For this review, take the finished solid that the model builds, in its own axes (mm). Face numbers are marked on the shaded views. A direction names the side the tool comes from. Round coordinates to 2 decimals unless told otherwise and drop trailing zeros. Loops run counter-clockwise (first coordinate to the right, second up) from the corner with the lowest first, then second, coordinate; pieces in that order, holes last.
1. Consider section A-A on y = -58.5. State the section outline as (x, z) points (3 decimals), then the cut area to 3 significant figures.
2. Tool access review of the marked faces 1 and 2: name each direction out of +Z, -Z, +X, -X, +Y, -Y from which nothing blocks a thin tool from reaching the whole face with its end or side.
3. Consider section C-C on x = 459.5. State the section outline as (y, z) points (3 decimals), then the cut area to 3 significant figures.
4. To check wall thickness, follow line 1 along Z through (x, y) = (-461.5, 75.5) (3 decimals); line 2 along Y through (x, z) = (544.5, -871.5) (3 decimals); line 3 along X through (y, z) = (135.5, -721) (3 decimals). State the ranges of each line that lie inside material, in increasing order.
5. Draft analysis for pull direction Z (two halves, no side actions). For the marked faces 3, 4 and 5, state which applies: released by +Z, released by -Z, zero draft, split by the parting line, or undercut.
6. Consider section B-B on z = -630. State the section outline as (x, y) points (3 decimals), then the cut area to 3 significant figures.
7. Clearance check with a flat-ended pin moving along its axis: pin 1 Ø10 at (x, z) = (-451.5, -403.5) entering from -Y (3 decimals). State where the tip first meets the part, or that it passes through.
Autodesk Inventor part; units mm, degrees
ref_plane "YZ Plane" through (0, 0, 0) normal (1, 0, 0) x (0, 1, 0)
ref_plane "XZ Plane" through (0, 0, 0) normal (0, 1, 0) x (-1, 0, 0)
ref_plane "XY Plane" through (0, 0, 0) normal (0, 0, 1) x (1, 0, 0)
sketch "Sketch1" plane through (0, 0, 0) normal (0, 0, 1) x (1, 0, 0)
  line L0 (-749.3, -254) -> (749.3, -254)
  line L1 (749.3, -254) -> (749.3, 254)
  line L2 (749.3, 254) -> (-749.3, 254)
  line L3 (-749.3, 254) -> (-749.3, -254)
  line L4 (-749.3, -254) -> (749.3, 254) construction
  line L5 (749.3, -254) -> (-749.3, 254) construction
  point P0 (0, 0)
  dimension "d0" = 1498.6
  dimension "d1" = 508
extrude "Extrusion1" add sketch "Sketch1" against normal blind 965.2
shell "Shell1" thickness 3.175 removed faces 0
sketch "Sketch2" plane through (-749.3, -254, 0) normal (0, -1, 0) x (1, 0, 0)
  line L0 (0, 0) -> (1498.6, 0)
  line L1 (1498.6, -965.2) -> (0, -965.2)
  line L2 (3.175, -127) -> (1495.425, -127)
  line L3 (1495.425, -127) -> (1495.425, -838.2)
  line L4 (1495.425, -838.2) -> (3.175, -838.2)
  line L5 (3.175, -838.2) -> (3.175, -127)
  line L6 (3.175, -3.175) -> (3.175, -962.025)
  line L7 (1495.425, -3.175) -> (1495.425, -962.025)
  point P0 (749.3, 0)
  dimension "d5" = 127
  dimension "d6" = 127
extrude "Extrusion2" cut sketch "Sketch2" against normal blind 3.175
equation "\"d6\" = d5"
properties part number "box_middlegoal" material "Polycarbonate, Clear"
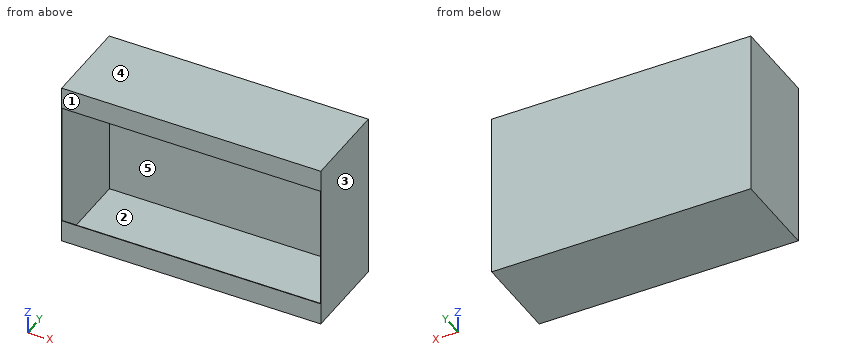
Resolved:
1. outline: (-749.3, -965.2) - (749.3, -965.2) - (749.3, 0) - (-749.3, 0) - close; hole (-746.125, -962.025) - (746.125, -962.025) - (746.125, -3.175) - (-746.125, -3.175) - close
1. area: 15,600 mm2
2. face 1: +Z, -Z, +X, -X, -Y
2. face 2: none
3. outline: (-254, -965.2) - (254, -965.2) - (254, 0) - (-254, 0) - (-254, -127) - (-250.825, -127) - (-250.825, -3.175) - (250.825, -3.175) - (250.825, -962.025) - (-250.825, -962.025) - (-250.825, -838.2) - (-254, -838.2) - close
3. area: 7,060 mm2
4. line 1: z = -965.2 to -962.025, -3.175 to 0
4. line 2: y = -254 to -250.825, 250.825 to 254
4. line 3: x = -749.3 to -746.125, 746.125 to 749.3
5. face 3: zero draft
5. face 4: released by +Z
5. face 5: undercut
6. outline: (-749.3, -254) - (-746.125, -254) - (-746.125, 250.825) - (746.125, 250.825) - (746.125, -254) - (749.3, -254) - (749.3, 254) - (-749.3, 254) - close
6. area: 7,960 mm2
7. pin 1: stops at y = 250.825
